Read the model definition and answer for the solid it produces. Units are mm, in the model's axes. A direction names the side the tool comes from. Give positions to 0.01 mm unless a question says otherwise; leave off trailing zeros. Loops run counter-clockwise (first coordinate to the right, second up) from the corner with the lowest first, then second, coordinate; pieces in that order, holes last. Notation, with made-up numbers: (-16.75, 41) - (13.25, 41) arc R10 ccw to (13.25, 49) - close; hole circle Ø2 at (88, 11). An arc over 180 degrees is marked (long way). Write each question's results on one line, items separated by ' | '. Start each with the question number.
Q1. Find the intervals of material crossed by line 1 (Y direction, x = 40.35, z = 0); line 2 (X direction, y = 1, z = -13.25); line 3 (Y direction, x = -13, z = -20.5), in increasing order. Write a range as from..to.
Q2. The part is cut by section D-D, the plane z = 20.5. Write down the section's boundary in (x, y).
Q3. The part is cut by section B-B, the plane x = -36.5. Write down the section's boundary in (y, z).
Q4. The part is cut by section A-A, the plane z = 13.25. Write down the section's boundary in (x, y).
Q5. Determine the mould class of faces 4 (the cylindrical face through (41, 10, -4)), 5 (the flat face through (40, 4, 5)), 6 (the cylindrical face through (40.53, 5.29, 0.38)) for opening direction Z: +Z half, -Z half, draft (parallel to the pull), parting line (faces both ways), or undercut.
Q6. Given pin 1 (10 mm diameter, centred on x = 12, z = 10, fed in from -Y); pin 2 (10 mm diameter, centred on x = 28.5, z = -8, fed in from +Y); pin 3 (2.5 mm diameter, centred on x = 41.5, y = 4, fed in from -Z); pin 4 (1.5 mm diameter, centred on x = 41.5, y = 4, fed in from +Z), each flat-ended and moving along its own axis, determine where each tip first touches the part or whether it passes through.
Q7. The part is cut by section C-C, the plane y = 3. Write down the section's boundary in (x, z).
Q8. For faces 1 (the flat face through (38, 5, 0)), 2 (the flat face through (40, 4, -5)), 3 (the cylindrical face through (-33.773, 1.014, -13.608)), determine the directions among +Z, -Z, +X, -X, +Y, -Y from which every point of the face is accessible in a straight line to the end or side of a thin tool.
```python
from build123d import *

# Parameters (mm, degrees)
SKETCH1_W           = 86
SKETCH1_H           = 46
BOSS_EXTRUDE1_DEPTH = 2
CUT_EXTRUDE1_REACH  = 50.806
SKETCH2_R           = 2.75
SKETCH3_W           = 5
SKETCH3_H           = 10
BOSS_EXTRUDE2_DEPTH = 10
SKETCH4_R           = 1.75
CUT_EXTRUDE2_DEPTH  = 10
FILLET1_R           = 5


with BuildPart() as part:
    # Sketch1 → Boss-Extrude1 (new body)
    with BuildSketch(Plane(origin=(0, 0, 0), x_dir=(1, 0, 0), z_dir=(0, 1, 0))):
        Rectangle(SKETCH1_W, SKETCH1_H)
    extrude(amount=BOSS_EXTRUDE1_DEPTH)

    # Sketch2 → Cut-Extrude1 (cut, up to next)
    with BuildSketch(Plane(origin=(0, 2, 0), x_dir=(1, 0, 0), z_dir=(0, 1, 0)), mode=Mode.PRIVATE) as cut_extrude1_sk1:
        with Locations(Location((-36.5, 13.25, 0), (0, 0, 270))):
            Circle(SKETCH2_R)
    cut_extrude1_tool1 = extrude(cut_extrude1_sk1.sketch, amount=-CUT_EXTRUDE1_REACH, mode=Mode.PRIVATE) & part.part
    # Sketch2 → Cut-Extrude1 (cut, up to next)
    with BuildSketch(Plane(origin=(0, 2, 0), x_dir=(1, 0, 0), z_dir=(0, 1, 0)), mode=Mode.PRIVATE) as cut_extrude1_sk2:
        with Locations(Location((-36.5, -13.25, 0), (0, 0, 270))):
            Circle(SKETCH2_R)
    cut_extrude1_tool2 = extrude(cut_extrude1_sk2.sketch, amount=-CUT_EXTRUDE1_REACH, mode=Mode.PRIVATE) & part.part
    add(cut_extrude1_tool1.solids().sort_by_distance((-36.5, 2, -13.25))[0], mode=Mode.SUBTRACT)
    add(cut_extrude1_tool2.solids().sort_by_distance((-36.5, 2, 13.25))[0], mode=Mode.SUBTRACT)

    # Sketch3 → Boss-Extrude2 (add)
    with BuildSketch(Plane(origin=(0, 2, 0), x_dir=(1, 0, 0), z_dir=(0, 1, 0))):
        with Locations((40.5, 0)):
            Rectangle(SKETCH3_W, SKETCH3_H)
    extrude(amount=BOSS_EXTRUDE2_DEPTH)

    # Sketch4 → Cut-Extrude2 (cut)
    with BuildSketch(Plane(origin=(43, 0, 0), x_dir=(0, 0, -1), z_dir=(1, 0, 0))):
        with Locations((0, 7)):
            Circle(SKETCH4_R)
    extrude(amount=-CUT_EXTRUDE2_DEPTH, mode=Mode.SUBTRACT)

    # Fillet1
    fillet1_edges = [part.edges().sort_by_distance(p)[0] for p in [
        (40.5, 12, -5),
        (40.5, 12, 5),
    ]]
    fillet(fillet1_edges, radius=FILLET1_R - 0.0001)  # a hair under: the kernel refuses the full size


solid = part.part
```
Check sheet entries:
1) line 1: y = 0..5.25, 8.75..12 | line 2: x = -43..-39.25, -33.75..43 | line 3: y = 0..2
2) outline: (-43, 0) - (43, 0) - (43, 2) - (-43, 2) - close
3) outline: (0, -23) - (2, -23) - (2, -16) - (0, -16) - close; (0, -10.5) - (2, -10.5) - (2, 10.5) - (0, 10.5) - close; (0, 16) - (2, 16) - (2, 23) - (0, 23) - close
4) outline: (-43, 0) - (-39.25, 0) - (-39.25, 2) - (-43, 2) - close; (-33.75, 0) - (43, 0) - (43, 2) - (-33.75, 2) - close
5) face 4: -Z half | face 5: +Z half | face 6: undercut
6) pin 1: stops at y = 0 | pin 2: stops at y = 2 | pin 3: stops at z = -5 | pin 4: stops at z = 5
7) outline: (38, -5) - (43, -5) - (43, 5) - (38, 5) - close
8) face 1: +Z, -Z, -X, +Y | face 2: -Z, +X, -X, +Y | face 3: +Y, -Y
